Source: CAD feature listing. Evaluate the final solid. Frame: model axes, mm. A direction names the side the tool comes from. Give positions to 0.01 mm unless a question says otherwise; leave off trailing zeros. Loops run counter-clockwise (first coordinate to the right, second up) from the corner with the lowest first, then second, coordinate; pieces in that order, holes last. Notation, with made-up numbers: M 89.5,66.5 L 107.5,66.5 A29 cw 107.5,99.5 Z; hole C 54.25,22.5 d11. An arc over 180 degrees is marked long. Write item = value, one per line.
from build123d import *

# Parameters (mm, degrees)
F0_R     = 1.6
F0_W     = 22
F0_H     = 20.2
F1_DEPTH = 7.2
F2_SIZE  = 2
F3_SIZE  = 1


with BuildPart() as f1:
    # F0 (on Top) → F1 (new body)
    with BuildSketch(Plane.XY):
        Polygon((13, 12.1), (-19.8, 12.1), (-19.8, 4.9), (-13, 4.9), (-13, -14.9), (13, -14.9), (13, -10.1), (13, -9.5), (19.4, -9.5), (19.4, -2.3), (13, -2.3), align=None)
        with Locations((15.8, -5.9)):
            Circle(F0_R, mode=Mode.SUBTRACT)
        with Locations((-16.2, 8.5)):
            Circle(F0_R, mode=Mode.SUBTRACT)
        Rectangle(F0_W, F0_H, mode=Mode.SUBTRACT)
    extrude(amount=F1_DEPTH)

    # F2
    f2_edges = [f1.edges().sort_by_distance(p)[0] for p in [
        (-19.8, 4.9, 3.6),
        (-19.8, 12.1, 3.6),
        (19.4, -9.5, 3.6),
        (19.4, -2.3, 3.6),
    ]]
    chamfer(f2_edges, length=F2_SIZE)

    # F3
    f3_edges = [f1.edges().sort_by_distance(p)[0] for p in [
        (11, 10.1, 3.6),
        (-11, 10.1, 3.6),
        (-11, -10.1, 3.6),
        (11, -10.1, 3.6),
    ]]
    chamfer(f3_edges, length=F3_SIZE)


solid = f1.part
1. Cut plane A-A, the plane x = 15.8. Return the cut outline in (y, z).
Derived:
outline = M -9.5,0 L -7.5,0 L -7.5,7.2 L -9.5,7.2 Z; M -4.3,0 L -2.3,0 L -2.3,7.2 L -4.3,7.2 Z
2. First-contact query: pin 1 Ø2 at (y, z) = (-11.5, 6.5) entering from -X; pin 2 Ø1.5 at (y, z) = (6, 1.5) entering from -X; pin 3 Ø1.6 at (y, z) = (-11.5, 4.5) entering from +X. Flat tips, straight axial feed; report the tip coordinate or a pass-through.
Derived:
pin_1 = -13
pin_2 = -19.65
pin_3 = 13
3. Cut plane B-B, the plane y = 8.5. Return the cut outline in (x, z).
Derived:
outline = M -19.8,0 L -17.8,0 L -17.8,7.2 L -19.8,7.2 Z; M -14.6,0 L -11,0 L -11,7.2 L -14.6,7.2 Z; M 11,0 L 13,0 L 13,7.2 L 11,7.2 Z
4. Cut plane C-C, the plane z = 5.5. Return the cut outline in (x, y), then the cut area to 3 significant figures.
Derived:
outline = M -19.8,6.9 L -17.8,4.9 L -13,4.9 L -13,-14.9 L 13,-14.9 L 13,-9.5 L 17.4,-9.5 L 19.4,-7.5 L 19.4,-4.3 L 17.4,-2.3 L 13,-2.3 L 13,12.1 L -17.8,12.1 L -19.8,10.1 Z; hole C -16.2,8.5 d3.2; hole M -11,-9.1 L -10,-10.1 L 10,-10.1 L 11,-9.1 L 11,9.1 L 10,10.1 L -10,10.1 L -11,9.1 Z; hole C 15.8,-5.9 d3.2
area = 331 mm²
5. Material intervals for probe 1 along X at (y, z) = (-6, 3); probe 2 along Y at (x, z) = (-2, 4.25); probe 3 along X at (y, z) = (0.5, 6.75), sorted ascending. Write a range as from..to.
Derived:
probe_1 = -13..-11, 11..14.2, 17.4..19.4
probe_2 = -14.9..-10.1, 10.1..12.1
probe_3 = -13..-11, 11..13
6. Pull-direction query (Y, two-part tool) for faces 4 (the flat face through (18.4, -3.3, 3.5)), 5 (the flat face through (10.5, 9.6, 3.5)), 6 (the flat face through (13, 5, 4)); classes: +Y half, -Y half, draft (parallel to the pull), parting line (faces both ways), or undercut.
Derived:
face_4 = +Y half
face_5 = undercut
face_6 = draft
7. Reachability of faces 1 (the flat face through (15, -2.3, 4)), 2 (the flat face through (13, -12, 4)), 3 (the flat face through (-10.5, -9.6, 3.5)) from +Z, -Z, +X, -X, +Y, -Y: full face, straight path, thin tool, end or side. Return the list, or none.
Derived:
face_1 = +Z, -Z, +X, +Y
face_2 = +Z, -Z, +X, -Y
face_3 = +Z, -Z
8. Cut plane D-D, the plane y = 2.75. Return the cut outline in (x, z).
Derived:
outline = M -13,0 L -11,0 L -11,7.2 L -13,7.2 Z; M 11,0 L 13,0 L 13,7.2 L 11,7.2 Z
